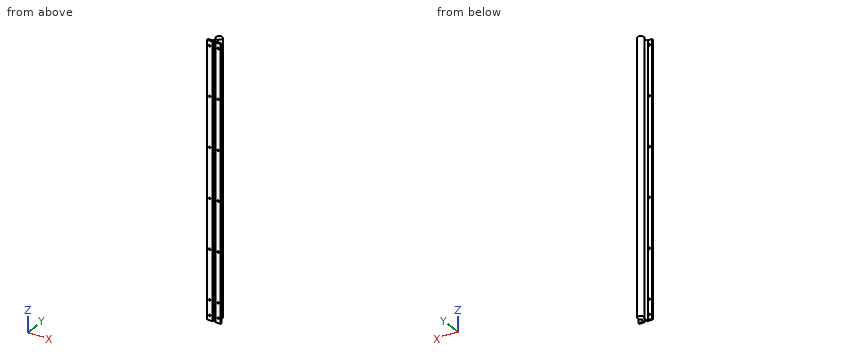
```python
from build123d import *

# Parameters (mm, degrees)
SKETCH1_R               = 12.5
BOSS_EXTRUDE1_DEPTH     = 1100
CHAMFER1_SIZE           = 1
SKETCH2_R               = 3.3
CUT_EXTRUDE1_DEPTH      = 40.5
CUT_EXTRUDE1_DEPTH_BACK = 7


with BuildPart() as part:
    # Sketch1 → Boss-Extrude1 (new body)
    with BuildSketch(Plane.XY):
        with Locations((0, 33)):
            Circle(SKETCH1_R)
        Polygon((-27.5, 0), (-4.75, 0), (-4.75, 6.5), (4.75, 6.5), (4.75, 0), (27.5, 0), (27.5, 6), (10.75, 6), (2.089745962, 21), (-2.089745962, 21), (-10.75, 6), (-27.5, 6), align=None)
    extrude(amount=-BOSS_EXTRUDE1_DEPTH)

    # Chamfer1
    chamfer1_edges = [part.edges().sort_by_distance(p)[0] for p in [
        (4.75, 0, -550),
        (-4.75, 0, -550),
    ]]
    chamfer(chamfer1_edges, length=CHAMFER1_SIZE)

    # Sketch2 → Cut-Extrude1 (cut, two sides)
    with BuildSketch(Plane(origin=(0, 6, 0), x_dir=(1, 0, 0), z_dir=(0, 1, 0))) as cut_extrude1_sk:
        with Locations((17.5, 20)):
            Circle(SKETCH2_R)
        with Locations((-17.5, 20)):
            Circle(SKETCH2_R)
        with Locations((-17.5, 220)):
            Circle(SKETCH2_R)
        with Locations((17.5, 220)):
            Circle(SKETCH2_R)
        with Locations((-17.5, 420)):
            Circle(SKETCH2_R)
        with Locations((17.5, 420)):
            Circle(SKETCH2_R)
        with Locations((-17.5, 620)):
            Circle(SKETCH2_R)
        with Locations((17.5, 620)):
            Circle(SKETCH2_R)
        with Locations((-17.5, 820)):
            Circle(SKETCH2_R)
        with Locations((17.5, 820)):
            Circle(SKETCH2_R)
        with Locations((-17.5, 1020)):
            Circle(SKETCH2_R)
        with Locations((17.5, 1020)):
            Circle(SKETCH2_R)
        with Locations((-17.5, 1220)):
            Circle(SKETCH2_R)
        with Locations((17.5, 1220)):
            Circle(SKETCH2_R)
        with Locations((-17.5, 1420)):
            Circle(SKETCH2_R)
        with Locations((17.5, 1420)):
            Circle(SKETCH2_R)
        with Locations((-17.5, 1620)):
            Circle(SKETCH2_R)
        with Locations((17.5, 1620)):
            Circle(SKETCH2_R)
        with Locations((17.5, 1080)):
            Circle(SKETCH2_R)
        with Locations((-17.5, 1080)):
            Circle(SKETCH2_R)
    extrude(amount=CUT_EXTRUDE1_DEPTH, mode=Mode.SUBTRACT)
    extrude(cut_extrude1_sk.sketch, amount=-CUT_EXTRUDE1_DEPTH_BACK, mode=Mode.SUBTRACT)


solid = part.part
```
Can you work these out from the model? Positions are in its coordinate system, mm. Coordinates: 2 decimals unless noted, no trailing zeros. Order: outer loops, then holes, each group sorted by start corner. A loop starts at its lowest first (then second) coordinate and runs counter-clockwise, first axis right, second up.
1. If we section it at A-A (z = -165): Please give me the cut outline in (x, y), then the cut area to 3 significant figures.
2. I need wall thicknesses on line 1 (X direction, y = 1.3, z = -820); line 2 (X direction, y = 3, z = -524); line 3 (Y direction, x = 21, z = -382.5). Which ranges of each line are inside material? Lowest first, please.
3. I'm going to push flat-ended pins straight in: pin 1 (8.5 mm diameter, centred on x = 17.5, z = -820, fed in from +Y); pin 2 (13.5 mm diameter, centred on x = 18, z = -775.5, fed in from +Y); pin 3 (2 mm diameter, centred on y = 22.5, z = -165, fed in from -X). Where does each tip first touch, or does it pass through?
4. If we section it at B-B (y = 33): Please give me the cut outline in (x, z).
Entries:
1. outline: (-27.5, 0) - (-5.75, 0) - (-4.75, 1) - (-4.75, 6.5) - (4.75, 6.5) - (4.75, 1) - (5.75, 0) - (27.5, 0) - (27.5, 6) - (10.75, 6) - (2.26, 20.71) arc R12.5 ccw (long way) to (-2.26, 20.71) - (-10.75, 6) - (-27.5, 6) - close
1. area: 949 mm2
2. line 1: x = -27.5 to -20.8, -14.2 to -4.75, 4.75 to 14.2, 20.8 to 27.5
2. line 2: x = -27.5 to -4.75, 4.75 to 27.5
2. line 3: y = 0 to 6
3. pin 1: stops at y = 6
3. pin 2: stops at y = 38.45
3. pin 3: stops at x = -8.12
4. outline: (-12.5, -1100) - (12.5, -1100) - (12.5, 0) - (-12.5, 0) - close
